The model under review builds one solid part; all positions refer to its coordinate system, in mm. Face numbers are marked on the shaded views. Give positions to 0.01 mm unless a question says otherwise; leave off trailing zeros. Order: outer loops, then holes, each group sorted by start corner. A loop starts at its lowest first (then second) coordinate and runs counter-clockwise, first axis right, second up. Notation, with made-up numbers: (17, 66) -> (63, 66) arc R10 cw to (63, 83) -> close; hole circle Ø10 at (56, 80.5). An arc over 180 degrees is marked (long way). Use one line per item in the form item = value.
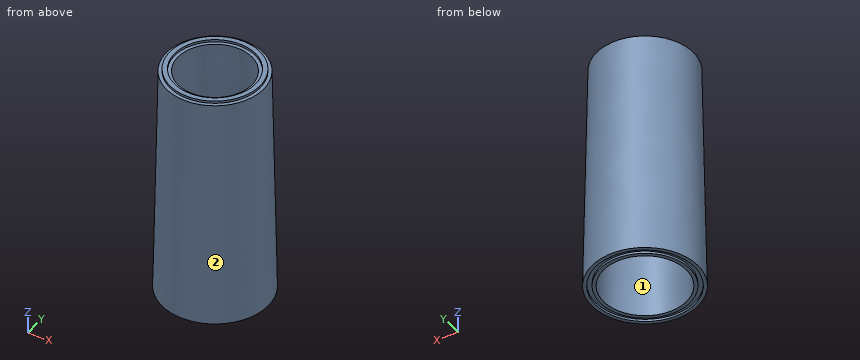
```python
from build123d import *

# Parameters (mm, degrees)
F0_W = 2
F0_H = 1


with BuildPart() as f1:
    # F0 (on Front) → F1 (revolve)
    with BuildSketch(Plane.XZ):
        Polygon((16, 100), (18, 0), (19.5, 0), (19.5, 1), (21.5, 1), (21.5, 0), (23, 0), (21, 100), (19.5, 100), (17.5, 100), align=None)
        with Locations((18.5, 100.5)):
            Rectangle(F0_W, F0_H)
    revolve(axis=Axis((0, 0, 83.813059), (0, 0, 1)))

    # F0 (on Front) → F2 (revolve, cut)
    with BuildSketch(Plane.XZ):
        with Locations((20.5, 0.5)):
            Rectangle(F0_W, F0_H)
    revolve(axis=Axis((0, 0, 83.813059), (0, 0, 1)), mode=Mode.SUBTRACT)


solid = f1.part
```
1. Add section B-B on z = 14. Give the boundary of the cut face in (x, y), then the cut area to 3 significant figures.
Values:
outline = circle Ø45.44 at (0, 0); hole circle Ø35.44 at (0, 0)
area = 635 mm^2
2. For L1, parallel to Y at x = 0, z = 100.4; L2, parallel to X at y = -16, z = 21; L3, parallel to X at y = -13, z = 54.5, list the stretches that pass through material, from the lowest coordinate up.
Values:
L1 = -19.5 to -17.5, 17.5 to 19.5
L2 = -15.93 to -7.28, 7.28 to 15.93
L3 = -17.64 to -10.81, 10.81 to 17.64
3. Add section A-A on z = 38. Give the boundary of the cut face in (x, y).
Values:
outline = circle Ø44.48 at (0, 0); hole circle Ø34.48 at (0, 0)
4. For pin 1 Ø4 at (x, y) = (-15, -17) entering from +Z; pin 2 Ø12 at (x, z) = (14, 72) entering from -Y; pin 3 Ø1.5 at (x, z) = (-6.5, 54) entering from +Y, all flat-tipped, find the tip position at first contact; note any pin that passes through.
Values:
pin_1 = 100
pin_2 = -20.02
pin_3 = 21.15
5. The part is to be moulded in two halves that separate along Y. For the marked faces 1 and 2, say which applies: +Y half, -Y half, draft (parallel to the pull), parting line (faces both ways), or undercut.
Values:
face_1 = undercut
face_2 = parting line
